Geometry check sheet. Reference: the model listing, model coordinates, mm. Face numbers are marked on the shaded views. Round coordinates to 2 decimals unless told otherwise and drop trailing zeros. Write each loop counter-clockwise with the first axis right and the second up, starting at its lowest first coordinate (ties: lowest second). Pieces come first, ordered by that corner, then holes. Notation, with made-up numbers: M 32.5,-8 L 55.5,-8 A22 cw 55.5,31 Z; hole C 39.25,68 d5. An arc over 180 degrees is marked long. Use a Markdown table: item, result.
Autodesk Inventor part; units mm, degrees
ref_plane "YZ Plane" through (0, 0, 0) normal (1, 0, 0) x (0, 1, 0)
ref_plane "XZ Plane" through (0, 0, 0) normal (0, 1, 0) x (-1, 0, 0)
ref_plane "XY Plane" through (0, 0, 0) normal (0, 0, 1) x (1, 0, 0)
sketch "Sketch1" plane through (0, 0, 0) normal (0, 1, 0) x (-1, 0, 0)
  circle A0 centre (0, 0) radius 75
  dimension "d0" = 150
extrude "Extrusion1" add sketch "Sketch1" along normal blind 10
sketch "Sketch2" plane through (0, 10, 0) normal (0, 1, 0) x (1, 0, 0)
  circle A0 centre (0, 0) radius 17.5
  dimension "d5" = 35
extrude "Extrusion2" cut sketch "Sketch2" against normal blind 10
sketch "Sketch3" plane through (0, 10, 0) normal (0, 1, 0) x (1, 0, 0)
  circle A0 centre (0, 0) radius 40
  dimension "d8" = 80
extrude "Extrusion3" cut sketch "Sketch3" against normal blind 5
fillet "Fillet2" radius 5 1 edges at (-17.5, 5, 0)
sketch "Sketch5" plane through (0, 10, 0) normal (0, 1, 0) x (1, 0, 0)
  circle A0 centre (0, 0) radius 67.5 construction
  circle A1 centre (0, 67.5) radius 4
  dimension "d46" = 135
  dimension "d47" = 8
hole "Hole2" at (0, 10, -67.5) direction (0, -1, 0) diameter 8 end through all
pattern_circular "Circular Pattern2" count 8 over 360 about axis through (0, -10, 0) along (0, 1, 0) of "Hole2"
properties part number "faceplate" material "Stainless Steel"
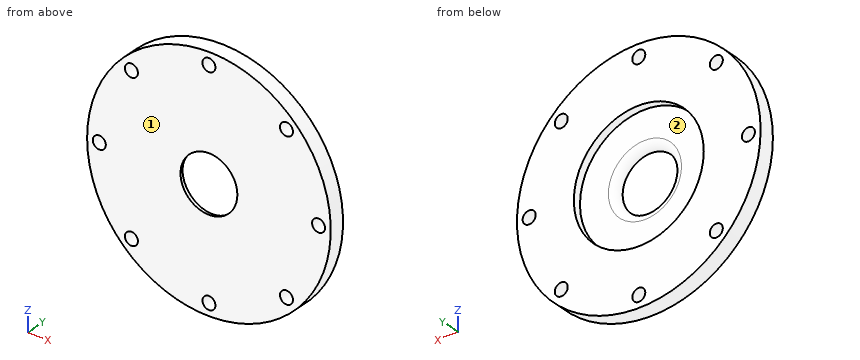
Item 1: Cross-section at C-C, the plane x = 67.5. Record the cut outline in (y, z), and give its area (3 significant figures).
Outcome:
| item | result |
|---|---|
| outline | M 0,-32.69 L 10,-32.69 L 10,-4 L 0,-4 Z; M 0,4 L 10,4 L 10,32.69 L 0,32.69 Z |
| area | 574 mm2 |
Item 2: Mould release check, pull along X, two halves, no side actions. Record for the marked faces 1 and 2: +X half, -X half, draft (parallel to the pull), parting line (faces both ways), or undercut.
Outcome:
| item | result |
|---|---|
| face 1 | draft |
| face 2 | undercut |
Item 3: Cross-section at A-A, the plane z = 0. Count the separate pieces of the cut face and the enclosed holes in it, and give its area (3 significant figures).
Outcome:
| item | result |
|---|---|
| separate pieces | 4 |
| enclosed holes | 0 |
| area | 754 mm2 |
Item 4: Cross-section at B-B, the plane z = -67.5. Record the cut outline in (x, y).
Outcome:
| item | result |
|---|---|
| outline | M -32.69,0 L -4,0 L -4,10 L -32.69,10 Z; M 4,0 L 32.69,0 L 32.69,10 L 4,10 Z |
Item 5: Go/stop test with flat-tipped pins: pin 1 (7 mm diameter, centred on x = 0, z = 67.5, fed in from +Y); pin 2 (3 mm diameter, centred on x = 30, y = 8, fed in from -Z); pin 3 (6 mm diameter, centred on x = -43, y = 3, fed in from +Z); pin 4 (1 mm diameter, centred on x = -7.5, y = 7.5, fed in from -Z). Record where each tip stops, or that it passes through.
Outcome:
| item | result |
|---|---|
| pin 1 | passes through |
| pin 2 | stops at z = -69.37 |
| pin 3 | stops at z = 63.44 |
| pin 4 | stops at z = -74.67 |
Item 6: Material ranges on line 1 along Z through (x, y) = (50.5, 6); line 2 along X through (y, z) = (8.75, -45); line 3 along Z through (x, y) = (-48, 9.75), recorded low to high. Write a range as from..to.
Outcome:
| item | result |
|---|---|
| line 1 | z = -55.45..-50.62, -44.84..44.84, 50.62..55.45 |
| line 2 | x = -60..-50.65, -44.81..44.81, 50.65..60 |
| line 3 | z = -57.63..-51.72, -43.74..43.74, 51.72..57.63 |
